```python
from build123d import *

# Parameters (mm, degrees)
PARED_START                = 21.5
SK_PARED_W                 = 50
SK_PARED_H                 = 63.3
PARED_DEPTH                = 6.35
CABEZA_START               = 21.5
SK_CABEZA_R                = 25
CABEZA_DEPTH               = 6.35
PASO_CUBO_J5_START         = 21.5
SK_PASO_CUBO_J5_R          = 18
PASO_CUBO_J5_DEPTH         = 6.35
PASANTE_M3_CINCHO_START    = 21.5
SK_PASANTE_M3_CINCHO_R     = 1.7
PASANTE_M3_CINCHO_DEPTH    = 6.35
SK_ROSCA_M3_DESDE_ABAJO_R  = 1.25
ROSCA_M3_DESDE_ABAJO_DEPTH = 9


with BuildPart() as part:
    # Sk_Pared → Pared (new body)
    with BuildSketch(Plane(origin=(0, 0, 0), x_dir=(1, 0, 0), z_dir=(0, 1, 0)).offset(PARED_START)):
        with Locations((0, -458)):
            Rectangle(SK_PARED_W, SK_PARED_H)
    extrude(amount=PARED_DEPTH)

    # Sk_Cabeza → Cabeza (add)
    with BuildSketch(Plane(origin=(0, 0, 0), x_dir=(1, 0, 0), z_dir=(0, 1, 0)).offset(CABEZA_START)):
        with Locations((0, -490)):
            Circle(SK_CABEZA_R)
    extrude(amount=CABEZA_DEPTH)

    # Sk_Paso_cubo_J5 → Paso_cubo_J5 (cut)
    with BuildSketch(Plane(origin=(0, 0, 0), x_dir=(1, 0, 0), z_dir=(0, 1, 0)).offset(PASO_CUBO_J5_START)):
        with Locations(Location((0, -490, 0), (0, 0, 270))):
            Circle(SK_PASO_CUBO_J5_R)
    extrude(amount=PASO_CUBO_J5_DEPTH, mode=Mode.SUBTRACT)

    # Sk_Pasante_M3_cincho → Pasante_M3_cincho (cut)
    with BuildSketch(Plane(origin=(0, 0, 0), x_dir=(1, 0, 0), z_dir=(0, 1, 0)).offset(PASANTE_M3_CINCHO_START)):
        with Locations(Location((-12, -455, 0), (0, 0, 270))):
            Circle(SK_PASANTE_M3_CINCHO_R)
    extrude(amount=PASANTE_M3_CINCHO_DEPTH, mode=Mode.SUBTRACT)

    # Sk_Rosca_M3_desde_abajo → Rosca_M3_desde_abajo (cut)
    with BuildSketch(Plane(origin=(0, 0, 426.35), x_dir=(-1, 0, 0), z_dir=(0, 0, -1))):
        with Locations((15, 24.675)):
            Circle(SK_ROSCA_M3_DESDE_ABAJO_R)
        with Locations((-15, 24.675)):
            Circle(SK_ROSCA_M3_DESDE_ABAJO_R)
    extrude(amount=-ROSCA_M3_DESDE_ABAJO_DEPTH, mode=Mode.SUBTRACT)


solid = part.part
```
The listing builds one solid part. Answer for the finished solid, in the listing's coordinates (mm). A direction names the side the tool comes from. Give positions to 0.01 mm unless a question says otherwise; leave off trailing zeros. Order: outer loops, then holes, each group sorted by start corner. A loop starts at its lowest first (then second) coordinate and runs counter-clockwise, first axis right, second up. Notation, with made-up numbers: (49, 22.5) -> (70, 22.5) arc R27 ccw to (70, 40.5) -> close; hole circle Ø10 at (60, -10.5). An arc over 180 degrees is marked (long way). Answer as a JSON object with one key per item and string values. Group by question number.
Item 1: A tool of negligible diameter and unlimited length cuts with its end or side. For faces 1 (the cylindrical face through (15.271, 23.455, 430.787)), 2 (the flat face through (-25, 25, 458)), from which of +Z, -Z, +X, -X, +Y, -Y can it reach the whole face along a straight path? Write none if from no direction.
Item 2: Consider L1, parallel to Y at x = 15, z = 433.25 (3 decimals); L2, parallel to X at y = 23.25, z = 490; L3, parallel to Z at x = -6, y = 24.25. Determine where each line is inside the solid, lowest interval first. Write a range as from..to.
Item 3: The part is cut by section D-D on x = 21. Write down the section's boundary in (y, z), and give its area (3 significant figures).
Item 4: The part is cut by section B-B on z = 455. Write down the section's boundary in (x, y).
Item 5: The part is cut by section C-C on x = -12. Write down the section's boundary in (y, z).
Item 6: The part is cut by section A-A on x = 0. Write down the section's boundary in (y, z), and give its area (3 significant figures).
Item 7: Determine the mould class of faces 3 (the cylindrical face through (-11.93, 24.63, 453.3)), 4 (the flat face through (15, 25, 435.35)), 5 (the cylindrical face through (-0.555, 24.631, 514.994)), 6 (the flat face through (0, 21.5, 460)) for opening direction X: pulls with the +X half, pulls with the -X half, needs draft (parallel to the pull), parting line crosses it, or undercut.
Item 8: Flat-ended cylindrical pins translate along their axes: pin 1 (2 mm diameter, centred on x = -15, y = 24.675, fed in from +Z); pin 2 (0.8 mm diameter, centred on x = 15.5, y = 25, fed in from -Z); pin 3 (3 mm diameter, centred on x = 15, y = 24.675, fed in from +Z). Find the tip coordinate at first contact, or state that the pin passes through.
Result set:
{
 "1": {"face 1": "-Z", "face 2": "+Z, -Z, -X, +Y, -Y"},
 "2": {"L1": "21.5..23.425, 25.925..27.85", "L2": "-25..-18, 18..25", "L3": "426.35..473.03, 506.97..514.27"},
 "3": {"outline": "(21.5, 426.35) -> (27.85, 426.35) -> (27.85, 503.56) -> (21.5, 503.56) -> close", "area": "490 mm²"},
 "4": {"outline": "(-25, 21.5) -> (-13.7, 21.5) -> (-13.7, 27.85) -> (-25, 27.85) -> close; (-10.3, 21.5) -> (25, 21.5) -> (25, 27.85) -> (-10.3, 27.85) -> close"},
 "5": {"outline": "(21.5, 426.35) -> (27.85, 426.35) -> (27.85, 453.3) -> (21.5, 453.3) -> close; (21.5, 456.7) -> (27.85, 456.7) -> (27.85, 476.58) -> (21.5, 476.58) -> close; (21.5, 503.42) -> (27.85, 503.42) -> (27.85, 511.93) -> (21.5, 511.93) -> close"},
 "6": {"outline": "(21.5, 426.35) -> (27.85, 426.35) -> (27.85, 472) -> (21.5, 472) -> close; (21.5, 508) -> (27.85, 508) -> (27.85, 515) -> (21.5, 515) -> close", "area": "334 mm²"},
 "7": {"face 3": "undercut", "face 4": "undercut", "face 5": "parting line crosses it", "face 6": "needs draft"},
 "8": {"pin 1": "z = 510.71", "pin 2": "z = 435.35", "pin 3": "z = 511.04"}
}
